```python
from build123d import *

# Parameters (mm, degrees)
SKETCH1_W           = 8
SKETCH1_H           = 4
BOSS_EXTRUDE1_DEPTH = 35
SKETCH2_R           = 1.8
CUT_EXTRUDE1_DEPTH  = 37.124783736
FILLET1_R           = 4


with BuildPart() as part:
    # Sketch1 → Boss-Extrude1 (new body)
    with BuildSketch(Plane.XY):
        with Locations((4, -2)):
            Rectangle(SKETCH1_W, SKETCH1_H)
    extrude(amount=BOSS_EXTRUDE1_DEPTH)

    # Sketch2 → Cut-Extrude1 (cut, through all)
    with BuildSketch(Plane(origin=(0, 0, 0), x_dir=(1, 0, 0), z_dir=(0, 1, 0))):
        with Locations(Location((4, -4, 0), (0, 0, 270))):
            Circle(SKETCH2_R)
        with Locations(Location((4, -31, 0), (0, 0, 270))):
            Circle(SKETCH2_R)
    extrude(amount=-CUT_EXTRUDE1_DEPTH, mode=Mode.SUBTRACT)

    # Fillet1
    fillet1_edges = [part.edges().sort_by_distance(p)[0] for p in [
        (0, -2, 0),
        (8, -2, 0),
        (0, -2, 35),
        (8, -2, 35),
    ]]
    fillet(fillet1_edges, radius=FILLET1_R - 0.0001)  # a hair under: the kernel refuses the full size


solid = part.part
```
Geometry check sheet. Reference: the model listing, model coordinates, mm. Round coordinates to 2 decimals unless told otherwise and drop trailing zeros. Loops run counter-clockwise (first coordinate to the right, second up) from the corner with the lowest first, then second, coordinate; pieces in that order, holes last. Notation, with made-up numbers: M 15.25,87.25 L 49.25,87.25 A27 ccw 49.25,125.25 Z; hole C -9.75,14.25 d6. An arc over 180 degrees is marked long. Return JSON: item names as keys, results as strings. Group by question number.
(1) Section check A-A, the plane y = -0.9. Give the number of separate pieces and of enclosed holes in the cut face, and give its area (3 significant figures).
(2) Go/stop test with a flat-tipped pin: pin 1 (4.5 mm diameter, centred on x = 4, z = 31, fed in from -Y). Record where the tip stops, or that it passes through.
(3) Section check B-B, the plane x = 7.5. Enter the section's corners in (y, z), and give its area (3 significant figures).
(4) Scan lines: line 1 along X through (y, z) = (-1.1, 4); line 2 along Z through (x, y) = (5.25, -0.15); line 3 along Z through (x, y) = (3.5, -3). Record each from-to range of solid material in increasing order. Write a range as [from, to].
(5) Section check C-C, the plane x = 1.25. Enter the section's corners in (y, z).
(6) Mould release check, pull along Z, two halves, no side actions. Record for faces 1 (the face through (0, -2, 17)), 2 (the face through (6.797, -1.972, 1.141)), 3 (the face through (4.541, -1.972, 5.717)): pulls with the +Z half, pulls with the -Z half, needs draft (parallel to the pull), parting line crosses it, or undercut.
Data:
{
 "1": {"separate pieces": "1", "enclosed holes": "2", "area": "246 mm²"},
 "2": {"pin 1": "y = -4"},
 "3": {"outline": "M -4,2.06 L 0,2.06 L 0,32.94 L -4,32.94 Z", "area": "123 mm²"},
 "4": {"line 1": "[0, 2.2], [5.8, 8]", "line 2": "[0.2, 2.7], [5.3, 29.7], [32.3, 34.8]", "line 3": "[0.03, 2.27], [5.73, 29.27], [32.73, 34.97]"},
 "5": {"outline": "M -4,1.1 L 0,1.1 L 0,33.9 L -4,33.9 Z"},
 "6": {"face 1": "needs draft", "face 2": "pulls with the -Z half", "face 3": "undercut"}
}
